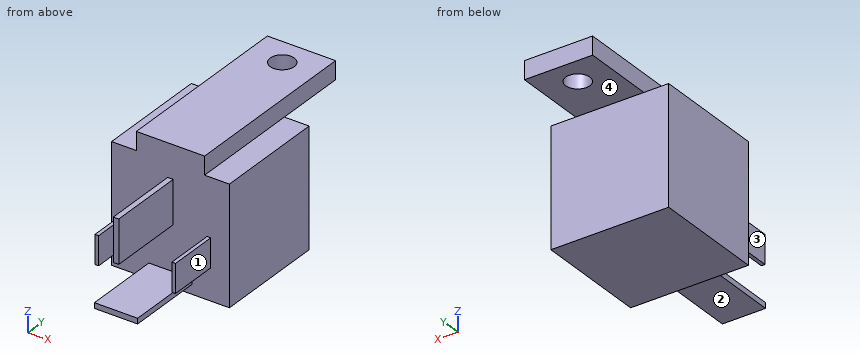
from build123d import *

# Parameters (mm, degrees)
SKETCH1_W           = 25.9
SKETCH1_H           = 25.9
BOSS_EXTRUDE1_DEPTH = 24.9
SKETCH2_W           = 15
SKETCH2_H           = 40.9
SKETCH2_R           = 2.65
BOSS_EXTRUDE2_DEPTH = 4
SKETCH3_W           = 9.5
SKETCH3_H           = 1.2
SKETCH3_W_2         = 0.8
SKETCH3_H_2         = 6.3
SKETCH3_W_3         = 1.2
SKETCH3_H_3         = 9.5
BOSS_EXTRUDE3_DEPTH = 11
SKETCH5_W           = 1.2
SKETCH5_H           = 9.5
SKETCH5_W_2         = 9.5
SKETCH5_H_2         = 1.2
BOSS_EXTRUDE4_DEPTH = 6


with BuildPart() as part:
    # Sketch1 → Boss-Extrude1 (new body)
    with BuildSketch(Plane(origin=(0, 0, 0), x_dir=(1, 0, 0), z_dir=(0, 1, 0))):
        with Locations((12.95, 12.95)):
            Rectangle(SKETCH1_W, SKETCH1_H)
    extrude(amount=BOSS_EXTRUDE1_DEPTH)

    # Sketch2 → Boss-Extrude2 (add)
    with BuildSketch(Plane.XY):
        with Locations((12.95, 20.45)):
            Rectangle(SKETCH2_W, SKETCH2_H)
        with Locations((12.95, 34.9)):
            Circle(SKETCH2_R, mode=Mode.SUBTRACT)
    extrude(amount=BOSS_EXTRUDE2_DEPTH)

    # Sketch3 → Boss-Extrude3 (add)
    with BuildSketch(Plane.XZ):
        with Locations((12.95, -23.2)):
            Rectangle(SKETCH3_W, SKETCH3_H)
        with Locations((21.4, -15.8)):
            Rectangle(SKETCH3_W_2, SKETCH3_H_2)
        with Locations((4.5, -15.8)):
            Rectangle(SKETCH3_W_2, SKETCH3_H_2)
        with Locations((12.95, -8)):
            Rectangle(SKETCH3_W_3, SKETCH3_H_3)
    extrude(amount=BOSS_EXTRUDE3_DEPTH)

    # Sketch5 → Boss-Extrude4 (add)
    with BuildSketch(Plane.XZ.offset(11)):
        with Locations((12.95, -8)):
            Rectangle(SKETCH5_W, SKETCH5_H)
        with Locations((12.95, -23.2)):
            Rectangle(SKETCH5_W_2, SKETCH5_H_2)
    extrude(amount=BOSS_EXTRUDE4_DEPTH)


solid = part.part
Source: CAD feature listing. Evaluate the final solid. Frame: model axes, mm. Face numbers are marked on the shaded views. A direction names the side the tool comes from. Give positions to 0.01 mm unless a question says otherwise; leave off trailing zeros. Order: outer loops, then holes, each group sorted by start corner. A loop starts at its lowest first (then second) coordinate and runs counter-clockwise, first axis right, second up. Notation, with made-up numbers: (-38, 77) -> (20, 77) arc R4 cw to (20, 83) -> close; hole circle Ø8 at (-10, -19.75). An arc over 180 degrees is marked (long way). Use a Markdown table: item, result.
1) Section query B-B, the plane x = 12.95. Return the cut outline in (y, z), then the cut area to 3 significant figures.
Answer list:
| item | result |
|---|---|
| outline | (-17, -23.8) -> (0, -23.8) -> (0, -25.9) -> (24.9, -25.9) -> (24.9, 0) -> (32.25, 0) -> (32.25, 4) -> (0, 4) -> (0, -3.25) -> (-17, -3.25) -> (-17, -12.75) -> (0, -12.75) -> (0, -22.6) -> (-17, -22.6) -> close; (37.55, 0) -> (40.9, 0) -> (40.9, 4) -> (37.55, 4) -> close |
| area | 969 mm² |
2) Contact query for flat-ended pins moving along their axis: P1, Ø3, axis at y = -8, z = -17.5, coming from the -X side; P2, Ø5, axis at y = 4.5, z = -6.5, coming from the -X side; P3, Ø1.9, axis at y = -4.5, z = -16.5, coming from the +X side; P4, Ø4.5, axis at x = 24.5, y = 11, coming from the +Z side. Output: stop coordinate, or through.
Answer list:
| item | result |
|---|---|
| P1 | x = 4.1 |
| P2 | x = 0 |
| P3 | x = 21.8 |
| P4 | z = 0 |
3) Section query C-C, the plane y = 34.9. Return the cut outline in (x, z), then the cut area to 3 significant figures.
Answer list:
| item | result |
|---|---|
| outline | (5.45, 0) -> (10.3, 0) -> (10.3, 4) -> (5.45, 4) -> close; (15.6, 0) -> (20.45, 0) -> (20.45, 4) -> (15.6, 4) -> close |
| area | 38.8 mm² |
4) Reachability of the marked faces 1, 2, 3 and 4 from +Z, -Z, +X, -X, +Y, -Y: full face, straight path, thin tool, end or side. Return the list, or none.
Answer list:
| item | result |
|---|---|
| face 1 | +Z, -Z, +X, -Y |
| face 2 | -Z, +X, -X, -Y |
| face 3 | +Z, -Z, -X, -Y |
| face 4 | -Z, +X, -X, +Y |
5) Ray query, line 1 along Y through (x, z) = (12.95, 2); line 2 along Y through (x, z) = (20, -13.75); line 3 along Z through (x, y) = (16, 37.5). Return the intervals inside material, ascending. Write a range as [from, to].
Answer list:
| item | result |
|---|---|
| line 1 | [0, 32.25], [37.55, 40.9] |
| line 2 | [0, 24.9] |
| line 3 | [0, 4] |
6) Section query D-D, the plane z = -14.75. Return the cut outline in (x, y).
Answer list:
| item | result |
|---|---|
| outline | (0, 0) -> (4.1, 0) -> (4.1, -11) -> (4.9, -11) -> (4.9, 0) -> (21, 0) -> (21, -11) -> (21.8, -11) -> (21.8, 0) -> (25.9, 0) -> (25.9, 24.9) -> (0, 24.9) -> close |
7) Section query A-A, the plane y = -9. Return the cut outline in (x, z).
Answer list:
| item | result |
|---|---|
| outline | (4.1, -18.95) -> (4.9, -18.95) -> (4.9, -12.65) -> (4.1, -12.65) -> close; (8.2, -23.8) -> (17.7, -23.8) -> (17.7, -22.6) -> (8.2, -22.6) -> close; (12.35, -12.75) -> (13.55, -12.75) -> (13.55, -3.25) -> (12.35, -3.25) -> close; (21, -18.95) -> (21.8, -18.95) -> (21.8, -12.65) -> (21, -12.65) -> close |
